```python
from build123d import *

# Parameters (mm, degrees)
BOSS_EXTRUDE1_DEPTH      = 5
BOSS_EXTRUDE1_DEPTH_BACK = 5
SKETCH1_R                = 1.5
CUT_EXTRUDE1_DEPTH       = 5
SKETCH3_W                = 7
SKETCH3_H                = 9
BOSS_EXTRUDE2_DEPTH      = 5


with BuildPart() as part:
    # Sketch1 → Boss-Extrude1 (new, two sides: drawn at the far end of the back side and taken through both)
    with BuildSketch(Plane(origin=(0, 0, 0), x_dir=(1, 0, 0), z_dir=(0, 1, 0)).offset(-BOSS_EXTRUDE1_DEPTH_BACK)):
        with BuildLine():
            Line((0, 22.5), (0, 36))
            Line((0, 36), (-36, 36))
            Line((-36, 36), (-36, -36))
            Line((-36, -36), (0, -36))
            Line((0, -36), (0, -22.5))
            ThreePointArc((0, -22.5), (-22.5, 0), (0, 22.5))
        make_face()
        with Locations(Location((-24.748737342, -24.748737342, 0), (0, 0, 270))):
            Circle(SKETCH1_R, mode=Mode.SUBTRACT)
        with Locations(Location((-24.748737342, 24.748737342, 0), (0, 0, 270))):
            Circle(SKETCH1_R, mode=Mode.SUBTRACT)
    extrude(amount=BOSS_EXTRUDE1_DEPTH + BOSS_EXTRUDE1_DEPTH_BACK)

    # Sketch2 → Cut-Extrude1 (cut)
    with BuildSketch(Plane(origin=(0, 5, 0), x_dir=(1, 0, 0), z_dir=(0, 1, 0))):
        Polygon((-23.161024101, 27.498737342), (-26.336450582, 27.498737342), (-27.924163822, 24.748737342), (-26.336450582, 21.998737342), (-23.161024101, 21.998737342), (-21.573310861, 24.748737342), align=None)
    cut_extrude1 = extrude(amount=-CUT_EXTRUDE1_DEPTH, mode=Mode.SUBTRACT)

    # Mirror1: Cut-Extrude1 across plane
    add(cut_extrude1.mirror(Plane.XY), mode=Mode.SUBTRACT)

    # Sketch3 → Boss-Extrude2 (add)
    with BuildSketch(Plane(origin=(0, 5, 0), x_dir=(1, 0, 0), z_dir=(0, 1, 0))):
        with Locations((3.5, -29.25)):
            Rectangle(SKETCH3_W, SKETCH3_H)
    boss_extrude2 = extrude(amount=-BOSS_EXTRUDE2_DEPTH)

    # Mirror2: Boss-Extrude2 across plane
    add(boss_extrude2.mirror(Plane.XY))


solid = part.part
```
Build history of the part. All positions in model axes, mm. A direction names the side the tool comes from. Give positions to 0.01 mm unless a question says otherwise; leave off trailing zeros. Loops run counter-clockwise (first coordinate to the right, second up) from the corner with the lowest first, then second, coordinate; pieces in that order, holes last.
Item 1: Slice it at C-C, the plane y = 3.5. List the corners of the cut face in (x, z), and give its area (3 significant figures).
Answers follow:
outline: (-36, -36) - (0, -36) - (0, -33.75) - (7, -33.75) - (7, -24.75) - (0, -24.75) - (0, -22.5) arc R22.5 cw to (0, 22.5) - (0, 24.75) - (7, 24.75) - (7, 33.75) - (0, 33.75) - (0, 36) - (-36, 36) - close; hole (-27.92, -24.75) - (-26.34, -27.5) - (-23.16, -27.5) - (-21.57, -24.75) - (-23.16, -22) - (-26.34, -22) - close; hole (-27.92, 24.75) - (-26.34, 22) - (-23.16, 22) - (-21.57, 24.75) - (-23.16, 27.5) - (-26.34, 27.5) - close
area: 1,870 mm2
Item 2: Flat gauge pins, fed straight in: pin 1 (5.5 mm diameter, centred on x = 2.5, z = -30.5, fed in from -Y); pin 2 (4 mm diameter, centred on x = 4.5, y = 3.5, fed in from -Z); pin 3 (2.5 mm diameter, centred on x = 5, y = 2, fed in from +Z). Where does each tip first touch, or does it go through?
Answers follow:
pin 1: stops at y = -5
pin 2: stops at z = -33.75
pin 3: stops at z = 33.75
Item 3: Pull direction Z, two halves, no side cores. Call faces 4 (the face through (7, 3, -29)), 5 (the face through (-18, 0, 36)), 6 (the face through (-18, 0, -36)), 7 (the face through (-22.38, 2.54, -23.35)): released by +Z, released by -Z, zero draft, split by the parting line, or undercut.
Answers follow:
face 4: zero draft
face 5: released by +Z
face 6: released by -Z
face 7: undercut
Item 4: Drill centre lines: line 1 (Z direction, x = 4, y = 1.25); line 2 (X direction, y = 3.25, z = 24.5); line 3 (Z direction, x = -7, y = 1.5). Where is each one in solid material? Low to high.
Answers follow:
line 1: z = -33.75 to -24.75, 24.75 to 33.75
line 2: x = -36 to -27.78, -21.72 to 0
line 3: z = -36 to -21.38, 21.38 to 36
Item 5: Slice it at D-D, the plane z = 0. List the corners of the cut face in (x, y).
Answers follow:
outline: (-36, -5) - (-22.5, -5) - (-22.5, 5) - (-36, 5) - close
Item 6: Slice it at A-A, the plane x = 1. List the corners of the cut face in (y, z), and give its area (3 significant figures).
Answers follow:
outline: (0, -33.75) - (5, -33.75) - (5, -24.75) - (0, -24.75) - close; (0, 24.75) - (5, 24.75) - (5, 33.75) - (0, 33.75) - close
area: 90.0 mm2
Item 7: Which spindle directions (+Z, -Z, +X, -X, +Y, -Y) get a long thin tool onto all of the face, cutting with end or side? Do faces 1 (the face through (3, 3, 24.75)), 2 (the face through (-25, 3, -21.999)), 3 (the face through (3, 3, -33.75)). Say none if no direction does.
Answers follow:
face 1: +X, +Y, -Y
face 2: +Y
face 3: -Z, +X, +Y, -Y
Item 8: Slice it at B-B, the plane y = -3.25. List the corners of the cut face in (x, z), and give its area (3 significant figures).
Answers follow:
outline: (-36, -36) - (0, -36) - (0, -22.5) arc R22.5 cw to (0, 22.5) - (0, 36) - (-36, 36) - close; hole circle Ø3 at (-24.75, -24.75); hole circle Ø3 at (-24.75, 24.75)
area: 1,780 mm2
